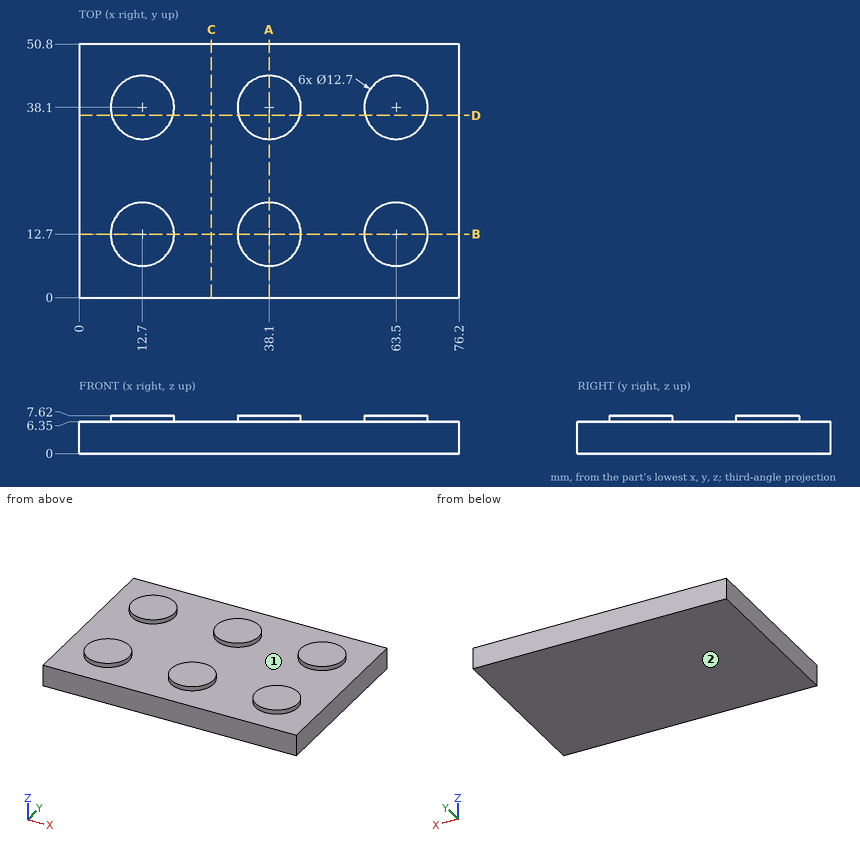
For this review, use the dimensioned drawing (mm, ordinates from the lowest corner) and the shaded views. Round coordinates to 2 decimals unless told otherwise and drop trailing zeros. Loops run counter-clockwise (first coordinate to the right, second up) from the corner with the lowest first, then second, coordinate; pieces in that order, holes last. Notation, with made-up numbers: (4.5, 38) -> (40.5, 38) arc R25 cw to (40.5, 62) -> close; hole circle Ø10 at (23, -12.75). An arc over 180 degrees is marked (long way). Write item = value, one per line. Start each with the question number.
Item 1: Take a section at B-B on y = 12.7. Give the boundary of the cut face in (x, z).
Item 2: To check wall thickness, follow L1, parallel to X at y = 39, z = 7.25; L2, parallel to Z at x = 57, y = 3.5; L3, parallel to Y at x = 38, z = 7. State the ranges of each line that lie inside material, in increasing order.
Item 3: Take a section at D-D on y = 36.5. Give the boundary of the cut face in (x, z).
Item 4: Mouldability with a two-part tool opening along X and no side actions: class the marked faces 1 and 2 as released by +X, released by -X, zero draft, split by the parting line, or undercut.
Item 5: Take a section at A-A on x = 38.1. Give the boundary of the cut face in (y, z).
Item 6: Insertion check: pin 1 (1 mm diameter, centred on x = 64, y = 12, fed in from -Z); pin 2 (1 mm diameter, centred on x = 31.5, y = 42, fed in from +Z). Each pin has a flat end and moves straight along its axis. Give the tip position at first contact, or say it passes through.
Item 7: Take a section at C-C on x = 26.5. Give the boundary of the cut face in (y, z), plus the area to 3 significant figures.
Result:
q1.outline = (0, 0) -> (76.2, 0) -> (76.2, 6.35) -> (69.85, 6.35) -> (69.85, 7.62) -> (57.15, 7.62) -> (57.15, 6.35) -> (44.45, 6.35) -> (44.45, 7.62) -> (31.75, 7.62) -> (31.75, 6.35) -> (19.05, 6.35) -> (19.05, 7.62) -> (6.35, 7.62) -> (6.35, 6.35) -> (0, 6.35) -> close
q2.L1 = 6.41 to 18.99, 31.81 to 44.39, 57.21 to 69.79
q2.L2 = 0 to 6.35
q2.L3 = 6.35 to 19.05, 31.75 to 44.45
q3.outline = (0, 0) -> (76.2, 0) -> (76.2, 6.35) -> (69.65, 6.35) -> (69.65, 7.62) -> (57.35, 7.62) -> (57.35, 6.35) -> (44.25, 6.35) -> (44.25, 7.62) -> (31.95, 7.62) -> (31.95, 6.35) -> (18.85, 6.35) -> (18.85, 7.62) -> (6.55, 7.62) -> (6.55, 6.35) -> (0, 6.35) -> close
q4.face_1 = undercut
q4.face_2 = zero draft
q5.outline = (0, 0) -> (50.8, 0) -> (50.8, 6.35) -> (44.45, 6.35) -> (44.45, 7.62) -> (31.75, 7.62) -> (31.75, 6.35) -> (19.05, 6.35) -> (19.05, 7.62) -> (6.35, 7.62) -> (6.35, 6.35) -> (0, 6.35) -> close
q6.pin_1 = 0
q6.pin_2 = 6.35
q7.outline = (0, 0) -> (50.8, 0) -> (50.8, 6.35) -> (0, 6.35) -> close
q7.area = 323 mm²
